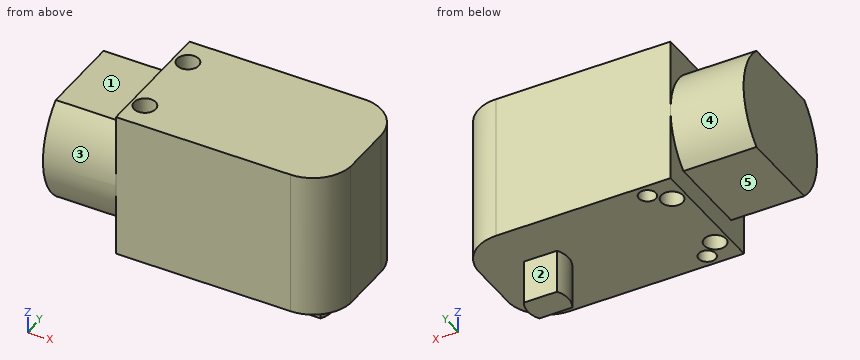
Autodesk Inventor part; units mm, degrees
ref_plane "YZ Plane" through (0, 0, 0) normal (1, 0, 0) x (0, 1, 0)
ref_plane "XZ Plane" through (0, 0, 0) normal (0, 1, 0) x (-1, 0, 0)
ref_plane "XY Plane" through (0, 0, 0) normal (0, 0, 1) x (1, 0, 0)
sketch "Sketch1" plane through (0, 0, 0) normal (0, 0, 1) x (1, 0, 0)
  line L0 (-18.0458, -12.2355) -> (12.3135, -12.2355)
  line L1 (19.1466, -5.9617) -> (19.1466, 3.4363)
  line L2 (12.2886, 10.2943) -> (-18.0458, 10.2943)
  line L3 (-18.0458, 10.2943) -> (-18.0458, -12.2355)
  line L4 (-18.0458, -12.2355) -> (16.3456, 11.0826) construction
  line L5 (18.0458, -10.2943) -> (-18.0458, 10.2943) construction
  arc A0 (19.1466, 3.4363) -> (12.2886, 10.2943) centre (12.2886, 3.4363) ccw
  arc A1 (12.3135, -12.2355) -> (19.1466, -5.9617) centre (12.3135, -5.3775) ccw
  point P0 (0, 0)
  point P1 (19.1466, -1.2627)
  dimension "d3" = 22.5298
  dimension "d10" = 9.398
  dimension "d11" = 6.858
  dimension "d12" = 6.858
extrude "Extrusion1" add sketch "Sketch1" along normal blind 25.4
sketch "Sketch2" plane through (0, 0, 0) normal (0, 0, -1) x (-1, 0, 0)
  line L0 (-12.2886, 10.2943) -> (18.0458, 10.2943)
  line L1 (18.0458, 10.2943) -> (18.0458, -12.2355)
  circle A0 centre (15.6074, 5.5191) radius 1.8796
  circle A1 centre (12.7451, 8.0337) radius 1.4732
  line L2 (-19.1466, -5.9617) -> (-19.1466, 3.4363)
  line L3 (18.0458, 10.2943) -> (18.0458, -12.2355)
  circle A2 centre (15.7097, -7.4978) radius 1.8796
  circle A3 centre (12.8872, -10.057) radius 1.4732
  point P0 (0, 0)
  dimension "d13" = 2.4384
  dimension "d14" = 4.7752
  dimension "d15" = 3.7592
  dimension "d16" = 2.9464
  dimension "d17" = 0.4572
  dimension "d18" = 2.2606
sketch "Sketch3" plane through (0, 0, 0) normal (0, 0, -1) x (-1, 0, 0)
  circle A0 centre (-9.0374, 0) radius 4.445
  line L0 (-19.1466, -5.9617) -> (-19.1466, 3.4363)
  line L1 (-6.1855, -2.3622) -> (-11.9313, -2.3622)
  line L2 (-6.1855, 2.3622) -> (-11.9313, 2.3622)
  arc A1 (-6.1855, -2.3622) -> (-6.1855, 2.3622) centre (-10.1887, 0) ccw
  arc A2 (-11.9313, 2.3622) -> (-11.9313, -2.3622) centre (-7.9281, 0) ccw
  line L3 (-5.5405, 0) -> (-12.5763, 0)
  line L4 (-9.0584, 2.3622) -> (-9.0584, -2.3622)
  point P0 (0, 0)
  dimension "d23" = 8.89
  dimension "d24" = 10.1092
  dimension "d45" = 4.7244
  dimension "d46" = 4.6482
  dimension "d47" = 4.6482
  dimension "d48" = 7.0358
sketch "Sketch4" plane through (-18.0458, -12.2355, 0) normal (-1, 0, 0) x (0, 0, 1)
  point P0 (0, 0)
  point P1 (25.4, 0)
  point P2 (0, 22.5298)
  point P3 (25.4, 22.5298)
extrude "Extrusion5" cut sketch "Sketch2" against normal blind 25.4 contours A2
extrude "Extrusion6" cut sketch "Sketch2" against normal blind 25.4 contours A0
extrude "Extrusion7" cut sketch "Sketch2" against normal blind 12.7 contours A1 | A3
sketch "Sketch5" plane through (-18.0458, -12.2355, 0) normal (-1, 0, 0) x (0, 0, 1)
  line L0 (25.4, 6.2738) -> (25.4, 15.6718)
  line L1 (0, 6.2738) -> (0, 15.6718)
  line L2 (0, 0) -> (25.4, 0)
  line L3 (12.7, 0) -> (12.7, 22.5298)
  line L4 (0, 22.5298) -> (25.4, 22.5298)
  line L5 (25.4, 0) -> (0, 22.5298)
  line L6 (25.4, 15.6718) -> (25.4, 22.5298)
  line L7 (0, 0) -> (25.4, 22.5298)
  line L8 (12.7, 3.937) -> (12.7, 18.5928) construction
  line L9 (21.6408, 3.937) -> (21.6408, 18.5928)
  line L10 (3.7592, 18.5928) -> (3.7592, 3.937)
  arc A0 (3.7592, 3.937) -> (21.6408, 3.937) centre (12.7, 12.1206) ccw
  arc A1 (21.6408, 18.5928) -> (3.7592, 18.5928) centre (12.7, 10.4092) ccw
  point P0 (0, 12.2355)
  point P1 (12.7, 11.2649)
  dimension "d39" = 22.5298
  dimension "d41" = 3.7592
extrude "Extrusion8" add sketch "Sketch5" along normal blind 12.7 contours A0 L7 L3 | L3 L5 A0 | A0 L10 A1 L5 L7 | L5 A1 L3 | L7 A1 L9 A0 L5 | L3 A1 L7
extrude "Extrusion9" add sketch "Sketch3" along normal blind 7.62 contours L1 L4 L3 A1 | L1 A2 L3 L4 | L3 L4 L2 A1 | L3 A2 L2 L4
properties part number "motor sumo jeffrey p"
Check sheet for the modelled part. Datum: model origin and axes. Units: mm. Face numbers are marked on the shaded views. A direction names the side the tool comes from. Round coordinates to 2 decimals unless told otherwise and drop trailing zeros. Loops run counter-clockwise (first coordinate to the right, second up) from the corner with the lowest first, then second, coordinate; pieces in that order, holes last.
1. Sectioned sample at D-D on y = 1.25. Record the boundary of the cut face in (x, z), and give its area (3 significant figures).
2. Sectioned sample at C-C on x = 9.5. Record the boundary of the cut face in (y, z).
3. Scan lines: probe 1 along Y at (x, z) = (-17, 21.5); probe 2 along Y at (x, z) = (9, -4); probe 3 along Z at (x, y) = (-5, 0.25). Record each from-to range of solid material in increasing order.
4. Set-up check for the marked faces 1, 2, 3, 4 and 5: record each of +Z, -Z, +X, -X, +Y, -Y from which the full face is reachable in a straight line by a thin tool's end or side.
5. Gauge pin test, flat ends, axial feed: pin 1 Ø3 at (x, y) = (-13, 8) entering from -Z; pin 2 Ø2.5 at (x, y) = (-12.89, -10.06) entering from -Z; pin 3 Ø1.7 at (x, z) = (8, -4) entering from -Y; pin 4 Ø2.5 at (x, y) = (-15.71, -7.5) entering from +Z. Record the tip position at first contact, or that the pin passes through.
6. Sectioned sample at B-B on z = 11.5. Record the boundary of the cut face in (x, y).
7. Sectioned sample at A-A on y = 4.5. Record the boundary of the cut face in (x, z), and give its area (3 significant figures).
Recorded:
1. outline: (-30.75, 3.76) - (-18.05, 3.76) - (-18.05, 0) - (5.71, 0) - (5.71, -7.62) - (12.41, -7.62) - (12.41, 0) - (19.15, 0) - (19.15, 25.4) - (-18.05, 25.4) - (-18.05, 21.64) - (-30.75, 21.64) - close
1. area: 1,220 mm2
2. outline: (-12.24, 0) - (-2.36, 0) - (-2.36, -7.62) - (2.36, -7.62) - (2.36, 0) - (10.29, 0) - (10.29, 25.4) - (-12.24, 25.4) - close
3. probe 1: y = -12.24 to -8.86, -6.13 to 4.26, 6.78 to 10.29
3. probe 2: y = -2.36 to 2.36
3. probe 3: z = 0 to 25.4
4. face 1: +Z, -X, +Y, -Y
4. face 2: -Z, +X, -X, +Y
4. face 3: -X, -Y
4. face 4: -X, +Y
4. face 5: -Z, -X, +Y, -Y
5. pin 1: stops at z = 0
5. pin 2: stops at z = 12.7
5. pin 3: stops at y = -2.36
5. pin 4: passes through
6. outline: (-30.75, -12.18) - (-18.05, -12.18) - (-18.05, -12.24) - (12.31, -12.24) arc R6.86 ccw to (19.15, -5.96) - (19.15, 3.44) arc R6.86 ccw to (12.29, 10.29) - (-18.05, 10.29) - (-18.05, 10.23) - (-30.75, 10.23) - close; hole circle Ø3.76 at (-15.71, -7.5); hole circle Ø3.76 at (-15.61, 5.52); hole circle Ø2.95 at (-12.89, -10.06); hole circle Ø2.95 at (-12.75, 8.03)
7. outline: (-30.75, 3.76) - (-18.05, 3.76) - (-18.05, 0) - (-17.19, 0) - (-17.19, 25.4) - (-18.05, 25.4) - (-18.05, 21.64) - (-30.75, 21.64) - close; (-14.03, 0) - (19.06, 0) - (19.06, 25.4) - (-14.03, 25.4) - close
7. area: 1,090 mm2
